Design review of the part shown in the three views and the two pictorial views. Dimensions are in mm from the part's minimum x, y and z. Round coordinates to 2 decimals unless told otherwise and drop trailing zeros. Order: outer loops, then holes, each group sorted by start corner. A loop starts at its lowest first (then second) coordinate and runs counter-clockwise, first axis right, second up. Notation, with made-up numbers: (42, 0.5) - (95, 0.5) arc R31 cw to (95, 36.5) - close; hole circle Ø9 at (40.25, 70). An arc over 180 degrees is marked (long way). One line per question, with ' | ' between items. Start each with the question number.
Item 1: Draft analysis for pull direction Z (two halves, no side actions). For the marked faces 1 and 2, state which applies: +Z half, -Z half, draft (parallel to the pull), parting line (faces both ways), or undercut.
Item 2: Add section A-A on z = 62.5. State the section outline as (x, y) points.
Item 3: For L1, parallel to Z at x = 64, y = 2.35; L2, parallel to Y at x = 101.5, z = 31; L3, parallel to Z at x = 83, y = 0.8, list the stretches that pass through material, from the lowest coordinate up. Write a range as [from, to].
Item 4: Insertion check: pin 1 Ø3 at (x, z) = (14.5, 62.5) entering from +Y; pin 2 Ø1.5 at (x, z) = (49, 24.5) entering from +Y; pin 3 Ø1 at (y, z) = (2, 69.5) entering from -X. Each pin has a flat end and moves straight along its axis. Give the tip position at first contact, or say it passes through.
Item 5: Add section B-B on x = 62.5. State the section outline as (y, z) points, and give its area (3 significant figures).
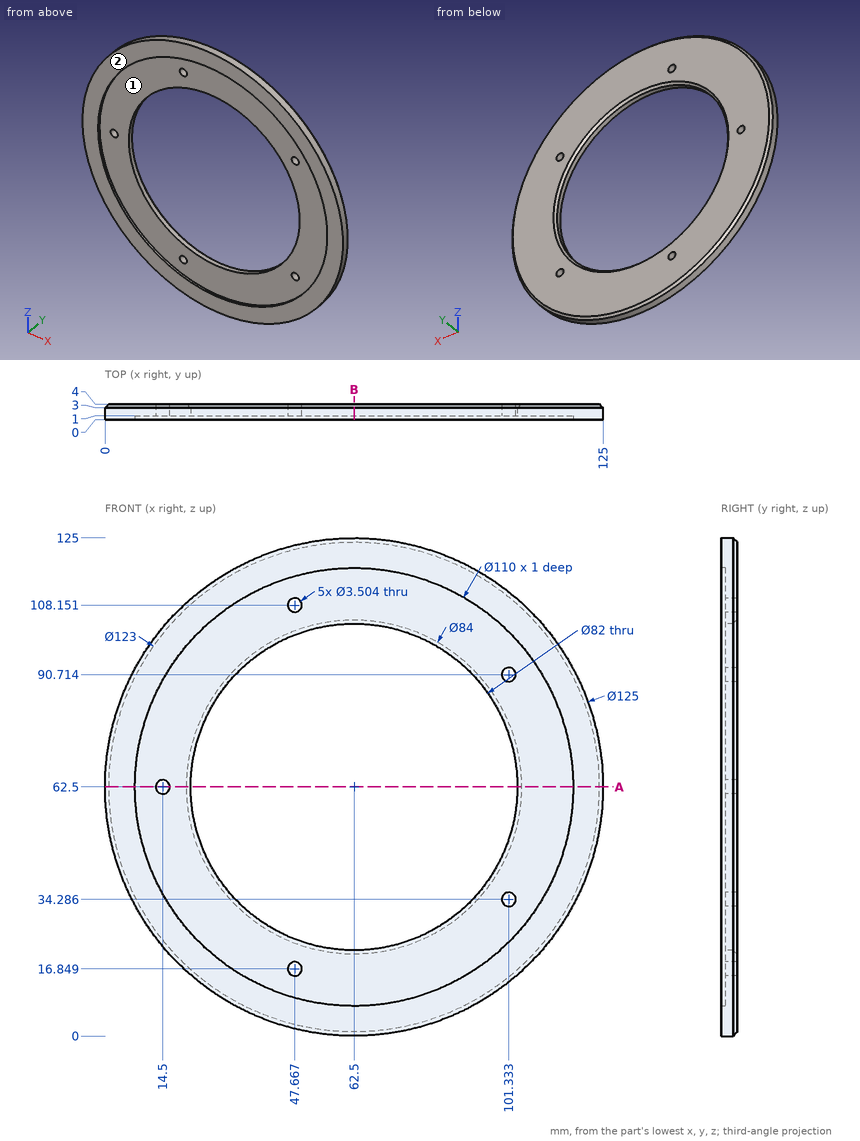
Determined:
1) face 1: undercut | face 2: draft
2) outline: (0, 0) - (7.5, 0) - (7.5, 1) - (12.75, 1) - (12.75, 4) - (1, 4) - (0, 3) - close; (16.25, 1) - (21.5, 1) - (21.5, 3) - (20.5, 4) - (16.25, 4) - close; (103.5, 1) - (117.5, 1) - (117.5, 0) - (125, 0) - (125, 3) - (124, 4) - (104.5, 4) - (103.5, 3) - close
3) L1: [0.02, 21.53], [103.47, 124.98] | L2: [1, 4] | L3: [3.46, 11.46], [113.54, 121.54]
4) pin 1: through | pin 2: y = 3.08 | pin 3: x = 0.34
5) outline: (0, 0) - (3, 0) - (4, 1) - (4, 20.5) - (3, 21.5) - (1, 21.5) - (1, 7.5) - (0, 7.5) - close; (0, 117.5) - (1, 117.5) - (1, 103.5) - (3, 103.5) - (4, 104.5) - (4, 124) - (3, 125) - (0, 125) - close | area: 142 mm2
